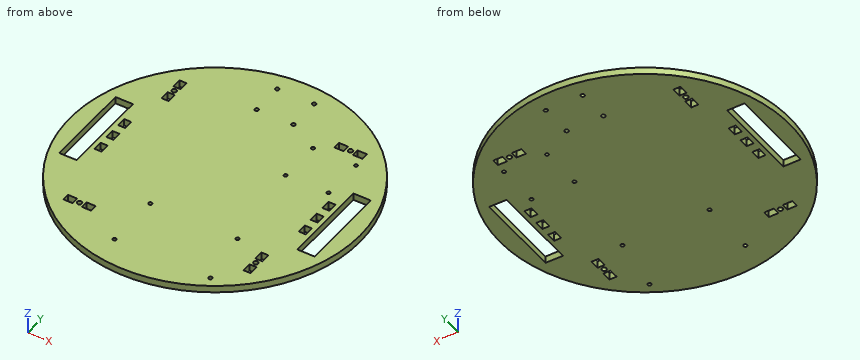
```python
from build123d import *

# Parameters (mm, degrees)
ESQUISSE1_R                  = 125
BOSS_EXTRU_1_DEPTH           = 6
ESQUISSE2_W                  = 15
ESQUISSE2_H                  = 76
ENL_V_MAT_EXTRU_1_DEPTH      = 7
ESQUISSE3_R                  = 2
ESQUISSE3_W                  = 8.2
ESQUISSE3_H                  = 6.2
ENL_V_MAT_EXTRU_2_DEPTH      = 7
R_P_TITION_CIRCULAIRE1_COUNT = 4
ESQUISSE4_W                  = 6.2
ESQUISSE4_H                  = 8.2
ENL_V_MAT_EXTRU_3_DEPTH      = 7
ESQUISSE7_R                  = 1.5621
ENL_V_MAT_EXTRU_6_DEPTH      = 6
ESQUISSE8_R                  = 1.5
ENL_V_MAT_EXTRU_7_DEPTH      = 10
ENL_V_MAT_EXTRU_8_REACH      = 8
ESQUISSE9_R                  = 1.65


with BuildPart() as part:
    # Esquisse1 → Boss.-Extru.1 (new body)
    with BuildSketch(Plane.XY):
        Circle(ESQUISSE1_R)
    extrude(amount=BOSS_EXTRU_1_DEPTH)

    # Esquisse2 → Enl_v. mat.-Extru.1 (cut, through all)
    with BuildSketch(Plane.XY.offset(6)):
        with Locations((-102.5, 0)):
            Rectangle(ESQUISSE2_W, ESQUISSE2_H)
    enl_v_mat_extru_1 = extrude(amount=-ENL_V_MAT_EXTRU_1_DEPTH, mode=Mode.SUBTRACT)

    # Sym_trie1: Enl_v. mat.-Extru.1 across plane
    add(enl_v_mat_extru_1.mirror(Plane(origin=(0, 0, 0), x_dir=(0, 0, 1), z_dir=(1, 0, 0))), mode=Mode.SUBTRACT)

    # Esquisse3 → Enl_v. mat.-Extru.2 (cut, through all)
    with BuildSketch(Plane(origin=(0, 0, 0), x_dir=(-1, 0, 0), z_dir=(0, 0, -1))):
        with Locations((-67, 78)):
            Circle(ESQUISSE3_R)
        with Locations((-75, 78)):
            Rectangle(ESQUISSE3_W, ESQUISSE3_H)
        with Locations((-59, 78)):
            Rectangle(ESQUISSE3_W, ESQUISSE3_H)
    enl_v_mat_extru_2 = extrude(amount=-ENL_V_MAT_EXTRU_2_DEPTH, mode=Mode.SUBTRACT)

    # R_p_tition circulaire1: Enl_v. mat.-Extru.2 ×4 about axis
    r_p_tition_circulaire1_axis = Axis((0, 0, 0), (0, 0, 1))
    for i in range(1, R_P_TITION_CIRCULAIRE1_COUNT):
        add(enl_v_mat_extru_2.rotate(r_p_tition_circulaire1_axis, i * 360 / R_P_TITION_CIRCULAIRE1_COUNT), mode=Mode.SUBTRACT)

    # Esquisse4 → Enl_v. mat.-Extru.3 (cut, through all)
    with BuildSketch(Plane(origin=(0, 0, 0), x_dir=(-1, 0, 0), z_dir=(0, 0, -1))):
        with Locations((88, 16)):
            Rectangle(ESQUISSE4_W, ESQUISSE4_H)
        with Locations((88, -16)):
            Rectangle(ESQUISSE4_W, ESQUISSE4_H)
        with Locations((88, 0)):
            Rectangle(ESQUISSE4_W, ESQUISSE4_H)
    enl_v_mat_extru_3 = extrude(amount=-ENL_V_MAT_EXTRU_3_DEPTH, mode=Mode.SUBTRACT)

    # Sym_trie2: Enl_v. mat.-Extru.3 across plane
    add(enl_v_mat_extru_3.mirror(Plane(origin=(0, 0, 0), x_dir=(0, 0, 1), z_dir=(1, 0, 0))), mode=Mode.SUBTRACT)

    # Esquisse7 → Enl_v. mat.-Extru.6 (cut)
    with BuildSketch(Plane(origin=(0, 0, 0), x_dir=(-1, 0, 0), z_dir=(0, 0, -1))):
        with Locations((23.116017499, -99.394574208)):
            Circle(ESQUISSE7_R)
        with Locations((23.116017499, -51.058374208)):
            Circle(ESQUISSE7_R)
        with Locations((-52.017182501, -51.058374208)):
            Circle(ESQUISSE7_R)
        with Locations((-59.510182501, -99.394574208)):
            Circle(ESQUISSE7_R)
    extrude(amount=-ENL_V_MAT_EXTRU_6_DEPTH, mode=Mode.SUBTRACT)

    # Esquisse8 → Enl_v. mat.-Extru.7 (cut)
    with BuildSketch(Plane(origin=(0, 0, 0), x_dir=(-1, 0, 0), z_dir=(0, 0, -1))):
        with Locations((-79.404950976, 65.925052584)):
            Circle(ESQUISSE8_R)
        with Locations((-42.404950976, 65.925052584)):
            Circle(ESQUISSE8_R)
        with Locations((-42.404950976, 28.925052584)):
            Circle(ESQUISSE8_R)
        with Locations((-79.404950976, 28.925052584)):
            Circle(ESQUISSE8_R)
    extrude(amount=-ENL_V_MAT_EXTRU_7_DEPTH, mode=Mode.SUBTRACT)

    # Esquisse9 → Enl_v. mat.-Extru.8 (cut, up to next)
    with BuildSketch(Plane.XY.offset(6), mode=Mode.PRIVATE) as enl_v_mat_extru_8_sk1:
        with Locations((-15.875, 108.97)):
            Circle(ESQUISSE9_R)
    enl_v_mat_extru_8_tool1 = extrude(enl_v_mat_extru_8_sk1.sketch, amount=-ENL_V_MAT_EXTRU_8_REACH, mode=Mode.PRIVATE) & part.part
    add(enl_v_mat_extru_8_tool1.solids().sort_by_distance((-15.875, 108.97, 6))[0], mode=Mode.SUBTRACT)
    # Esquisse9 → Enl_v. mat.-Extru.8 (cut, up to next)
    with BuildSketch(Plane.XY.offset(6), mode=Mode.PRIVATE) as enl_v_mat_extru_8_sk2:
        with Locations((15.875, 108.97)):
            Circle(ESQUISSE9_R)
    enl_v_mat_extru_8_tool2 = extrude(enl_v_mat_extru_8_sk2.sketch, amount=-ENL_V_MAT_EXTRU_8_REACH, mode=Mode.PRIVATE) & part.part
    add(enl_v_mat_extru_8_tool2.solids().sort_by_distance((15.875, 108.97, 6))[0], mode=Mode.SUBTRACT)
    # Esquisse9 → Enl_v. mat.-Extru.8 (cut, up to next)
    with BuildSketch(Plane.XY.offset(6), mode=Mode.PRIVATE) as enl_v_mat_extru_8_sk3:
        with Locations((15.875, 81.03)):
            Circle(ESQUISSE9_R)
    enl_v_mat_extru_8_tool3 = extrude(enl_v_mat_extru_8_sk3.sketch, amount=-ENL_V_MAT_EXTRU_8_REACH, mode=Mode.PRIVATE) & part.part
    add(enl_v_mat_extru_8_tool3.solids().sort_by_distance((15.875, 81.03, 6))[0], mode=Mode.SUBTRACT)
    # Esquisse9 → Enl_v. mat.-Extru.8 (cut, up to next)
    with BuildSketch(Plane.XY.offset(6), mode=Mode.PRIVATE) as enl_v_mat_extru_8_sk4:
        with Locations((-15.875, 81.03)):
            Circle(ESQUISSE9_R)
    enl_v_mat_extru_8_tool4 = extrude(enl_v_mat_extru_8_sk4.sketch, amount=-ENL_V_MAT_EXTRU_8_REACH, mode=Mode.PRIVATE) & part.part
    add(enl_v_mat_extru_8_tool4.solids().sort_by_distance((-15.875, 81.03, 6))[0], mode=Mode.SUBTRACT)


solid = part.part
```
Source: CAD feature listing. Evaluate the final solid. Frame: model axes, mm. Give positions to 0.01 mm unless a question says otherwise; leave off trailing zeros. Loops run counter-clockwise (first coordinate to the right, second up) from the corner with the lowest first, then second, coordinate; pieces in that order, holes last. Notation, with made-up numbers: (81.5, -28) -> (128.5, -28) arc R11 ccw to (128.5, -8) -> close; hole circle Ø4 at (1.5, -28). An arc over 180 degrees is marked (long way). Use a Markdown table: item, result. Add a question column.
(1) Section query C-C (y = -104.5). Output: boundary loops of the cut face in (x, z), then the cut area to 3 significant figures.
(2) Ray query, line 1 (Y direction, x = 16, z = 1.25); line 2 (X direction, y = -78.5, z = 0.95); line 3 (X direction, y = 75, z = 0.65). Return the intervals inside material, ascending.
(3) First-contact query: pin 1 Ø3 at (x, z) = (-51, 3) entering from +Y; pin 2 Ø3 at (x, z) = (87, 3.5) entering from +Y; pin 3 Ø1.8 at (y, z) = (77, 2.5) entering from -X; pin 4 Ø3 at (x, y) = (-23.12, -99.39) entering from +Z. Flat tips, straight axial feed; report the tip coordinate or a pass-through.
(4) Section query A-A (x = -45.5). Output: boundary loops of the cut face in (y, z).
(5) Section query B-B (z = 3.1). Count the separate pieces of the cut face and the enclosed holes in it, then the cut area to 3 significant figures.
Checked values:
| question | item | result |
|---|---|---|
| 1 | outline | (-68.59, 0) -> (68.59, 0) -> (68.59, 6) -> (-68.59, 6) -> close |
| 1 | area | 823 mm^2 |
| 2 | line 1 | -123.97 to 79.38, 82.68 to 107.32, 110.62 to 123.97 |
| 2 | line 2 | -97.28 to -79.1, -70.9 to -68.94, -65.06 to -63.1, -54.9 to 74.9, 81.1 to 97.28 |
| 2 | line 3 | -100 to -81.1, -74.9 to 54.9, 63.1 to 70.9, 79.1 to 100 |
| 3 | pin 1 | y = 114.78 |
| 3 | pin 2 | y = 91.19 |
| 3 | pin 3 | x = -99.17 |
| 3 | pin 4 | through |
| 4 | outline | (-116.42, 0) -> (116.42, 0) -> (116.42, 6) -> (-116.42, 6) -> close |
| 5 | separate pieces | 1 |
| 5 | enclosed holes | 32 |
| 5 | area | 46,000 mm^2 |
